```python
from build123d import *

# Parameters (mm, degrees)
SKETCH1_R           = 17.5
BOSS_EXTRUDE1_DEPTH = 18
SHELL1_T            = -2.3
SKETCH2_R           = 16.25
CUT_EXTRUDE1_DEPTH  = 1
SKETCH4_R           = 15.2
BOSS_EXTRUDE2_DEPTH = 6


with BuildPart() as part:
    # Sketch1 → Boss-Extrude1 (new body)
    with BuildSketch(Plane(origin=(0, 0, 0), x_dir=(1, 0, 0), z_dir=(0, 1, 0))):
        with Locations(Location((0, 0, 0), (0, 0, 270))):
            Circle(SKETCH1_R)
    extrude(amount=BOSS_EXTRUDE1_DEPTH)

    # Shell1
    shell1_openings = [part.faces().sort_by_distance(p)[0] for p in [
        (0, 18, 0),
    ]]
    offset(amount=SHELL1_T, openings=shell1_openings, kind=Kind.INTERSECTION)

    # Sketch2 → Cut-Extrude1 (cut)
    with BuildSketch(Plane(origin=(0, 18, 0), x_dir=(1, 0, 0), z_dir=(0, 1, 0))):
        with Locations(Location((0, 0, 0), (0, 0, 270))):
            Circle(SKETCH2_R)
    extrude(amount=-CUT_EXTRUDE1_DEPTH, mode=Mode.SUBTRACT)

    # Sketch4 → Boss-Extrude2 (add)
    with BuildSketch(Plane(origin=(0, 2.3, 0), x_dir=(1, 0, 0), z_dir=(0, 1, 0))):
        with Locations(Location((0, 0, 0), (0, 0, 270))):
            Circle(SKETCH4_R)
    extrude(amount=BOSS_EXTRUDE2_DEPTH)


solid = part.part
```
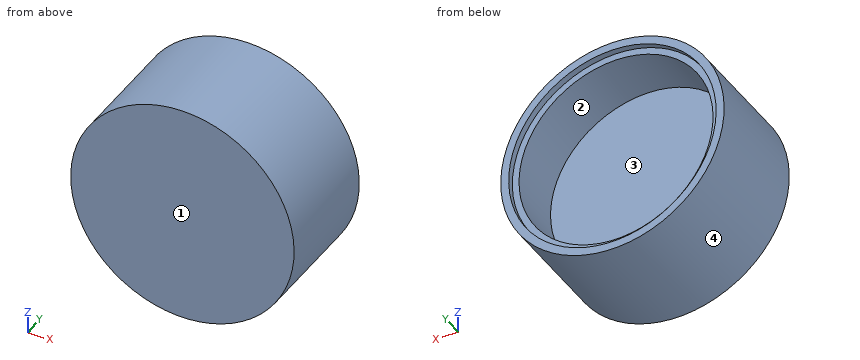
Can you work these out from the model? Positions are in its coordinate system, mm. Face numbers are marked on the shaded views. Round coordinates to 2 decimals unless told otherwise and drop trailing zeros. Loops run counter-clockwise (first coordinate to the right, second up) from the corner with the lowest first, then second, coordinate; pieces in that order, holes last. Notation, with made-up numbers: M 15.25,41 L 63.25,41 A10 ccw 63.25,46 Z; hole C 29.5,62.5 d5. An arc over 180 degrees is marked long. Answer in a Markdown table with one row per item.
1. Please list where these lines run through material, in increasing order: line 1 (X direction, y = 17.6, z = 0); line 2 (X direction, y = 12, z = 0); line 3 (Y direction, x = -12.5, z = 6.5). Write a range as from..to.
Established:
| item | result |
|---|---|
| line 1 | -17.5..-16.25, 16.25..17.5 |
| line 2 | -17.5..-15.2, 15.2..17.5 |
| line 3 | 0..8.3 |
2. If we section it at B-B, the plane z = 0: Please give me the cut outline in (x, y).
Established:
| item | result |
|---|---|
| outline | M -17.5,0 L 17.5,0 L 17.5,18 L 16.25,18 L 16.25,17 L 15.2,17 L 15.2,8.3 L -15.2,8.3 L -15.2,17 L -16.25,17 L -16.25,18 L -17.5,18 Z |
3. Thinking about a two-plate mould opening in Z: for the marked faces 1, 2, 3 and 4, which applies, pulls with the +Z half, pulls with the -Z half, needs draft (parallel to the pull), parting line crosses it, or undercut?
Established:
| item | result |
|---|---|
| face 1 | needs draft |
| face 2 | undercut |
| face 3 | undercut |
| face 4 | parting line crosses it |
4. I'm going to push flat-ended pins straight in: pin 1 Ø9 at (x, z) = (4, -6) entering from +Y; pin 2 Ø1 at (y, z) = (7, 11.5) entering from -X; pin 3 Ø2 at (x, y) = (2, 13.5) entering from +Z. Where does each tip first touch, or does it pass through?
Established:
| item | result |
|---|---|
| pin 1 | y = 8.3 |
| pin 2 | x = -13.61 |
| pin 3 | z = 17.47 |
5. If we section it at A-A, the plane x = 0: Please give me the cut outline in (y, z), plus the area to 3 significant figures.
Established:
| item | result |
|---|---|
| outline | M 0,-17.5 L 18,-17.5 L 18,-16.25 L 17,-16.25 L 17,-15.2 L 8.3,-15.2 L 8.3,15.2 L 17,15.2 L 17,16.25 L 18,16.25 L 18,17.5 L 0,17.5 Z |
| area | 333 mm² |
